Can you work these out from the model? Positions are in its coordinate system, mm. A direction names the side the tool comes from. Coordinates: 2 decimals unless noted, no trailing zeros. Write each loop counter-clockwise with the first axis right and the second up, starting at its lowest first coordinate (ties: lowest second). Pieces come first, ordered by that corner, then holes. Notation, with made-up numbers: (41, 75.25) - (94, 75.25) arc R13 ccw to (94, 100.25) - close; hole circle Ø11 at (-26.5, 63). An arc over 180 degrees is marked (long way). One line per question, with ' | ' between items. Start each with the question number.
from build123d import *

# Parameters (mm, degrees)
SALIENTE_EXTRUIR1_DEPTH = 175


with BuildPart() as part:
    # Croquis1 → Saliente-Extruir1 (new, symmetric)
    with BuildSketch(Plane.XY):
        with BuildLine():
            Line((5, 25), (22, 25))
            ThreePointArc((22, 25), (24.121320344, 24.121320344), (25, 22))
            Line((25, 22), (25, 5))
            Line((25, 5), (20, 5))
            Line((20, 5), (20, 12.464466094))
            Line((20, 12.464466094), (16, 12.464466094))
            Line((16, 12.464466094), (14, 10.464466094))
            Line((14, 10.464466094), (14, 0))
            Line((14, 0), (6, 0))
            Line((6, 0), (6, 5))
            Line((6, 5), (9, 5))
            Line((9, 5), (9, 9))
            Line((9, 9), (5, 9))
            Line((5, 9), (5, 6))
            Line((5, 6), (0, 6))
            Line((0, 6), (0, 14))
            Line((0, 14), (10.464466094, 14))
            Line((10.464466094, 14), (12.464466094, 16))
            Line((12.464466094, 16), (12.464466094, 20))
            Line((12.464466094, 20), (5, 20))
            Line((5, 20), (5, 25))
        make_face()
        Polygon((23.61230751, 18.478547627), (18.478547627, 23.61230751), (8.817158017, 23.61230751), (8.817158017, 22.328867539), (14.913358785, 22.328867539), (14.913358785, 18.359777384), (18.359777384, 14.913358785), (22.328867539, 14.913358785), (22.328867539, 8.817158017), (23.61230751, 8.817158017), align=None, mode=Mode.SUBTRACT)
    saliente_extruir1 = extrude(amount=SALIENTE_EXTRUIR1_DEPTH, both=True)

    # Simetría1: Saliente-Extruir1 across plane
    add(saliente_extruir1.mirror(Plane(origin=(0, 14, 175), x_dir=(0, 0, 1), z_dir=(1, 0, 0))))

    # Simetría7: part across plane


with BuildPart() as part_1:
    add(part.part)
    add(part.part.mirror(Plane(origin=(6, 0, 175), x_dir=(0, 0, 1), z_dir=(0, 1, 0))))


solid = part_1.part
(1) I'm going to push flat-ended pins straight in: pin 1 (2 mm diameter, centred on y = 1, z = -101.5, fed in from -X); pin 2 (6 mm diameter, centred on x = -19.5, y = 8.5, fed in from +Z); pin 3 (4 mm diameter, centred on x = -8.5, y = -17, fed in from +Z); pin 4 (3 mm diameter, centred on y = 0.5, z = -86.5, fed in from +X). Where does each tip first touch, or does it pass through?
(2) Which directions (+Z, -Z, +X, -X, +Y, -Y) give clear straight access to the entire face, cutting with the end or side of a thin tool? Please do faces 1 (the face through (-13, 25, 2)), 2 (the face through (23.612, -14, 2)).
(3) If we section it at A-A on x = 0.5: List the corners of the cut face in (y, z) for me.
(4) If we mould it in two halves opening along X, with no side actions, what happens to faces 3 (the face through (22.329, -12, 2)), 4 (the face through (25, 14, 2)), 5 (the face through (-23.612, -14, 2)), 6 (the face through (0, 11, 175))? For each: +X half, -X half, draft (parallel to the pull), parting line (faces both ways), or undercut.
(5) If I drill on probe 1 along X at (y, z) = (-13, 25); probe 2 along Y at (x, z) = (-8, -64), over which ranges is the centre line in solid material (lowest first)?
(6) If we section it at B-B on z = -98.5: Give the number of separate pieces and of enclosed holes in the cut face, plus the area to 3 significant figures.
Values:
1) pin 1: x = -14 | pin 2: z = 175 | pin 3: through | pin 4: x = 14
2) face 1: +Z, -Z, +X, -X, +Y | face 2: +Z, -Z
3) outline: (-14, -175) - (-6, -175) - (-6, 175) - (-14, 175) - close; (6, -175) - (14, -175) - (14, 175) - (6, 175) - close
4) face 3: undercut | face 4: +X half | face 5: undercut | face 6: draft
5) probe 1: -25 to -23.61, -22.33 to 22.33, 23.61 to 25 | probe 2: -25 to -20, -14 to -9, -5 to 5, 9 to 14, 20 to 25
6) separate pieces: 1 | enclosed holes: 5 | area: 1,220 mm2
